Build history of the part. All positions in model axes, mm. Face numbers are marked on the shaded views. A direction names the side the tool comes from. Give positions to 0.01 mm unless a question says otherwise; leave off trailing zeros. Order: outer loops, then holes, each group sorted by start corner. A loop starts at its lowest first (then second) coordinate and runs counter-clockwise, first axis right, second up. Notation, with made-up numbers: (35.5, 7.5) -> (88.5, 7.5) arc R13 cw to (88.5, 15.5) -> close; hole circle Ø6 at (31.25, -30.75). An arc over 180 degrees is marked (long way). Use a Markdown table: item, result. Add a question column.
```python
from build123d import *

# Parameters (mm, degrees)
CORTE_EXTRUS_O1_DEPTH = 32.287217837
PADR_OCIRCULAR2_COUNT = 9
CORTE_EXTRUS_O2_DEPTH = 32.134624111
ESBO_O7_W             = 0.2
ESBO_O7_H             = 30
CORTE_EXTRUS_O3_DEPTH = 10


with BuildPart() as part:
    # Esboço2 → Revolução1 (revolve)
    with BuildSketch(Plane.XY, mode=Mode.PRIVATE) as revolu_o1_sk:
        with BuildLine():
            Line((0, 0), (0, 16.464198342))
            ThreePointArc((0, 16.464198342), (0.321571182, 19.304004673), (1.27, 22))
            Line((1.27, 22), (2.03, 22))
            ThreePointArc((2.03, 22), (2.978428818, 19.304004673), (3.3, 16.464198342))
            Line((3.3, 16.464198342), (3.3, 0))
            Line((3.3, 0), (0, 0))
        make_face()
    revolve(revolu_o1_sk.sketch.rotate(Axis((0, 0, 0), (1, 0, 0)), 90), axis=Axis((0, 0, 0), (1, 0, 0)))

    # Esboço5 → Corte-extrusão1 (cut, through all)
    with BuildSketch(Plane(origin=(0, 0, 0), x_dir=(0, 0, -1), z_dir=(1, 0, 0))):
        with BuildLine():
            ThreePointArc((3.547062102, 16.950885739), (5.413227359, 19.685368366), (8.05493296, 21.680702805))
            ThreePointArc((8.05493296, 21.680702805), (0, 23.128657961), (-8.05493296, 21.680702805))
            ThreePointArc((-8.05493296, 21.680702805), (-5.413227359, 19.685368366), (-3.547062102, 16.950885739))
            ThreePointArc((-3.547062102, 16.950885739), (0, 14.691157961), (3.547062102, 16.950885739))
        make_face()
    corte_extrus_o1 = extrude(amount=CORTE_EXTRUS_O1_DEPTH, mode=Mode.SUBTRACT)

    # PadrãoCircular2: Corte-extrusão1 ×9 about axis
    padr_ocircular2_axis = Axis((0, 0, 0), (1, 0, 0))
    for i in range(1, PADR_OCIRCULAR2_COUNT):
        add(corte_extrus_o1.rotate(padr_ocircular2_axis, i * 360 / PADR_OCIRCULAR2_COUNT), mode=Mode.SUBTRACT)

    # Esboço6 → Corte-extrusão2 (cut, through all)
    with BuildSketch(Plane(origin=(3.3, 0, 0), x_dir=(0, 0, -1), z_dir=(1, 0, 0))):
        with BuildLine():
            Line((-2.236067977, 2), (2.236067977, 2))
            ThreePointArc((2.236067977, 2), (0, -3), (-2.236067977, 2))
        make_face()
    extrude(amount=-CORTE_EXTRUS_O2_DEPTH, mode=Mode.SUBTRACT)

    # Esboço7 → Corte-extrusão3 (cut)
    with BuildSketch(Plane(origin=(3.3, 0, 0), x_dir=(0, 0, -1), z_dir=(1, 0, 0))):
        with Locations((0, 17)):
            Rectangle(ESBO_O7_W, ESBO_O7_H)
    extrude(amount=-CORTE_EXTRUS_O3_DEPTH, mode=Mode.SUBTRACT)


solid = part.part
```
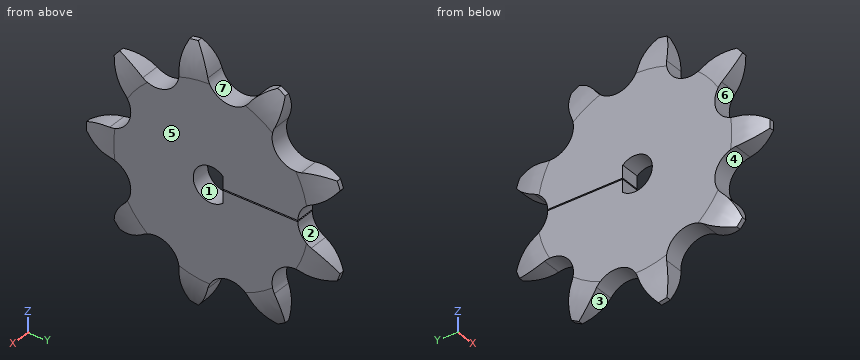
(1) Tool access for the marked faces 1, 2 and 3: list every direction of +Z, -Z, +X, -X, +Y, -Y with a clear straight run to the whole face (end or side of a thin tool).
(2) Band-saw the part on A-A on y = 3. Give the cut face in (x, z).
(3) Wall check: probe 1 along Z at (x, y) = (2.3, 0); probe 2 along Z at (x, y) = (2.45, 17); probe 3 along X at (y, z) = (10, -13.5). Give the ranges that are in metal, low to high.
(4) Band-saw the part on B-B on y = -8.5. Give the cut face in (x, z), plus the area to 3 significant figures.
(5) Mould opens along Z. For the marked faces 4, 5, 6 and 7 say: released by +Z, released by -Z, zero draft, split by the parting line, or undercut.
(6) Pin check, flat tips, straight feed: pin 1 Ø1 at (x, y) = (1.5, 7) entering from +Z; pin 2 Ø1.1 at (x, z) = (2, -1) entering from -Y. Stop position of each tip, or through.
Response:
| question | item | result |
|---|---|---|
| 1 | face 1 | +X, -X |
| 1 | face 2 | +X, -X, +Y |
| 1 | face 3 | -Z, +X, -X |
| 2 | outline | (0, -14.42) -> (3.3, -14.42) -> (3.3, -0.1) -> (0, -0.1) -> close; (0, 0.1) -> (3.3, 0.1) -> (3.3, 14.42) -> (0, 14.42) -> close |
| 3 | probe 1 | z = -16.11 to -3, 3 to 16.11 |
| 3 | probe 2 | z = -8.49 to -3.57, 3.57 to 8.49 |
| 3 | probe 3 | x = 0 to 3.3 |
| 4 | outline | (0, -12.28) -> (3.3, -12.28) -> (3.3, 12.28) -> (0, 12.28) -> close |
| 4 | area | 81.1 mm² |
| 5 | face 4 | undercut |
| 5 | face 5 | zero draft |
| 5 | face 6 | undercut |
| 5 | face 7 | released by +Z |
| 6 | pin 1 | stops at z = 17.36 |
| 6 | pin 2 | stops at y = -22 |
